Check sheet for the drawn part. Datum: minimum x, y, z corner. Units: mm. Give positions to 0.01 mm unless a question says otherwise; leave off trailing zeros. Write each loop counter-clockwise with the first axis right and the second up, starting at its lowest first coordinate (ties: lowest second). Pieces come first, ordered by that corner, then holes.
(1) Thickness scan on line 1 along X through (y, z) = (0.75, 5); line 2 along X through (y, z) = (0.3, 3.75); line 3 along X through (y, z) = (0.15, 2.5). Record the ranges inside material, lowest first.
(2) Cross-section at D-D (z = 5). Record the boundary of the cut face in (x, y), and give its area (3 significant figures).
(3) Cross-section at A-A (x = 7). Record the boundary of the cut face in (y, z).
(4) Cross-section at B-B (z = 3.5). Record the boundary of the cut face in (x, y), and give its area (3 significant figures).
(5) Cross-section at C-C (y = 1.1). Record the boundary of the cut face in (x, z).
(6) Depth check by flat-ended pin: P1, Ø5, axis at x = 7, z = 5, coming from the +Y side; P2, Ø3.5, axis at x = 34, z = 5, coming from the +Y side. Enter the tip coordinate at first touch or a pass-through.
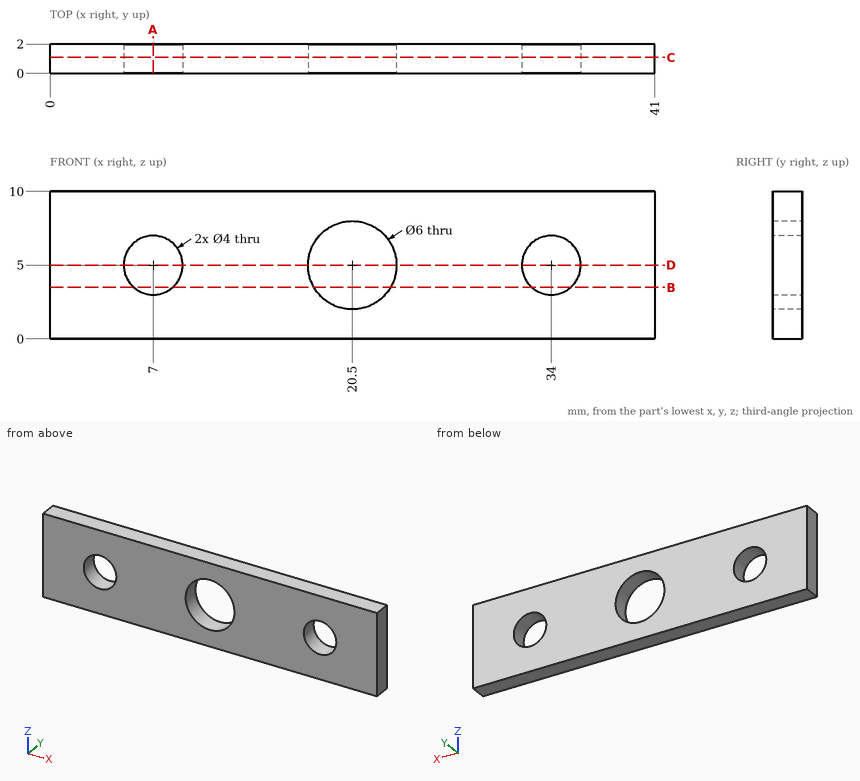
Reply:
1. line 1: x = 0 to 5, 9 to 17.5, 23.5 to 32, 36 to 41
1. line 2: x = 0 to 5.44, 8.56 to 17.77, 23.23 to 32.44, 35.56 to 41
1. line 3: x = 0 to 18.84, 22.16 to 41
2. outline: (0, 0) - (5, 0) - (5, 2) - (0, 2) - close; (9, 0) - (17.5, 0) - (17.5, 2) - (9, 2) - close; (23.5, 0) - (32, 0) - (32, 2) - (23.5, 2) - close; (36, 0) - (41, 0) - (41, 2) - (36, 2) - close
2. area: 54.0 mm2
3. outline: (0, 0) - (2, 0) - (2, 3) - (0, 3) - close; (0, 7) - (2, 7) - (2, 10) - (0, 10) - close
4. outline: (0, 0) - (5.68, 0) - (5.68, 2) - (0, 2) - close; (8.32, 0) - (17.9, 0) - (17.9, 2) - (8.32, 2) - close; (23.1, 0) - (32.68, 0) - (32.68, 2) - (23.1, 2) - close; (35.32, 0) - (41, 0) - (41, 2) - (35.32, 2) - close
4. area: 61.0 mm2
5. outline: (0, 0) - (41, 0) - (41, 10) - (0, 10) - close; hole circle Ø4 at (7, 5); hole circle Ø6 at (20.5, 5); hole circle Ø4 at (34, 5)
6. P1: stops at y = 2
6. P2: passes through
